For this review, take the finished solid that the model builds, in its own axes (mm). Face numbers are marked on the shaded views. A direction names the side the tool comes from. Coordinates: 2 decimals unless noted, no trailing zeros. Order: outer loops, then holes, each group sorted by start corner. A loop starts at its lowest first (then second) coordinate and runs counter-clockwise, first axis right, second up.
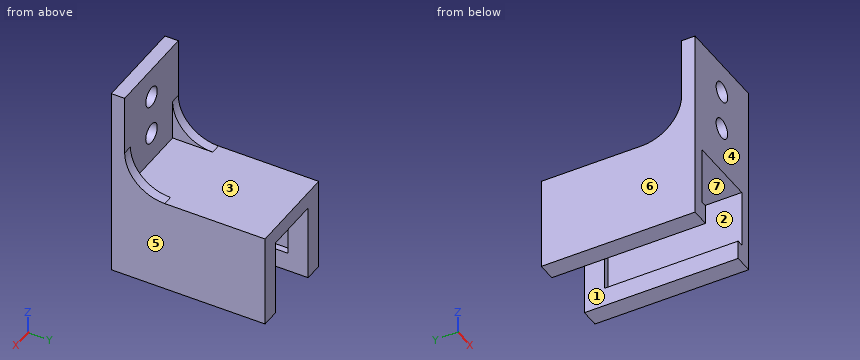
from build123d import *

# Parameters (mm, degrees)
SKETCH1_W           = 14
SKETCH1_H           = 23
BOSS_EXTRUDE1_DEPTH = 14
SKETCH2_W           = 10.4
SKETCH2_H           = 8.65
SKETCH2_W_2         = 8.5
SKETCH2_H_2         = 2.85
CUT_EXTRUDE1_DEPTH  = 20
SKETCH3_W           = 14
SKETCH3_H           = 15
SKETCH3_R           = 1.5
BOSS_EXTRUDE2_DEPTH = 2
BOSS_EXTRUDE3_DEPTH = 1.5
SKETCH5_W           = 8.5
SKETCH5_H           = 11.5
CUT_EXTRUDE2_DEPTH  = 4


with BuildPart() as part:
    # Sketch1 → Boss-Extrude1 (new body)
    with BuildSketch(Plane.XY):
        Rectangle(SKETCH1_W, SKETCH1_H)
    extrude(amount=BOSS_EXTRUDE1_DEPTH)

    # Sketch2 → Cut-Extrude1 (cut)
    with BuildSketch(Plane.XZ.offset(11.5)):
        with Locations((0, 7.175)):
            Rectangle(SKETCH2_W, SKETCH2_H)
        with Locations((0, 1.425)):
            Rectangle(SKETCH2_W_2, SKETCH2_H_2)
    extrude(amount=-CUT_EXTRUDE1_DEPTH, mode=Mode.SUBTRACT)

    # Sketch3 → Boss-Extrude2 (add)
    with BuildSketch(Plane.XZ.offset(11.5)):
        with Locations((0, 21.5)):
            Rectangle(SKETCH3_W, SKETCH3_H)
        with Locations((0, 18.5)):
            Circle(SKETCH3_R, mode=Mode.SUBTRACT)
        with Locations((0, 24.5)):
            Circle(SKETCH3_R, mode=Mode.SUBTRACT)
    extrude(amount=-BOSS_EXTRUDE2_DEPTH)

    # Sketch4 → Boss-Extrude3 (add)
    with BuildSketch(Plane.ZY.offset(7)):
        with BuildLine():
            Line((14, -3.5), (14, -9.5))
            Line((14, -9.5), (20, -9.5))
            ThreePointArc((20, -9.5), (15.757359313, -7.742640687), (14, -3.5))
        make_face()
    boss_extrude3 = extrude(amount=-BOSS_EXTRUDE3_DEPTH)

    # Mirror1: Boss-Extrude3 across plane
    add(boss_extrude3.mirror(Plane(origin=(0, 0, 0), x_dir=(0, 0, 1), z_dir=(1, 0, 0))))

    # Sketch5 → Cut-Extrude2 (cut, through all)
    with BuildSketch(Plane.XZ.offset(-8.5)):
        with Locations((0, 5.75)):
            Rectangle(SKETCH5_W, SKETCH5_H)
    extrude(amount=-CUT_EXTRUDE2_DEPTH, mode=Mode.SUBTRACT)


solid = part.part
1. Machinability: for the marked faces 1, 2, 3 and 4, which of the approach directions +Z, -Z, +X, -X, +Y, -Y give a long, thin tool a straight path to every point of the face, cutting with its end or side? Answer none if there is none.
Answer below:
face 1: -Z, +Y, -Y
face 2: -Y
face 3: +Z, +Y
face 4: +Z, -Z, +X, -X, -Y
2. Take a section at A-A, the plane x = 0. Give the boundary of the cut face in (y, z), plus the area to 3 significant figures.
Answer below:
outline: (-11.5, 11.5) - (11.5, 11.5) - (11.5, 14) - (-9.5, 14) - (-9.5, 17) - (-11.5, 17) - close; (-11.5, 20) - (-9.5, 20) - (-9.5, 23) - (-11.5, 23) - close; (-11.5, 26) - (-9.5, 26) - (-9.5, 29) - (-11.5, 29) - close
area: 75.5 mm2
3. Clearance check with flat-ended pins moving along their axes: pin 1 Ø1 at (x, z) = (-4.5, 5.5) entering from -Y; pin 2 Ø0.5 at (x, y) = (4.5, -4) entering from +Z; pin 3 Ø2.5 at (x, z) = (0, 18.5) entering from +Y; pin 4 Ø5 at (x, z) = (5, 18.5) entering from +Y. State where each tip first meets the part, or that it passes through.
Answer below:
pin 1: stops at y = 8.5
pin 2: stops at z = 14
pin 3: passes through
pin 4: stops at y = -8.02
4. Take a section at C-C, the plane y = -10. Give the boundary of the cut face in (x, z).
Answer below:
outline: (-7, 0) - (-4.25, 0) - (-4.25, 2.85) - (-5.2, 2.85) - (-5.2, 11.5) - (5.2, 11.5) - (5.2, 2.85) - (4.25, 2.85) - (4.25, 0) - (7, 0) - (7, 29) - (-7, 29) - close; hole circle Ø3 at (0, 18.5); hole circle Ø3 at (0, 24.5)
5. Take a section at B-B, the plane z = 24.5. Give the boundary of the cut face in (x, y).
Answer below:
outline: (-7, -11.5) - (-1.5, -11.5) - (-1.5, -9.5) - (-7, -9.5) - close; (1.5, -11.5) - (7, -11.5) - (7, -9.5) - (1.5, -9.5) - close
6. Take a section at D-D, the plane y = 1.25. Give the boundary of the cut face in (x, z), plus the area to 3 significant figures.
Answer below:
outline: (-7, 0) - (-4.25, 0) - (-4.25, 2.85) - (-5.2, 2.85) - (-5.2, 11.5) - (5.2, 11.5) - (5.2, 2.85) - (4.25, 2.85) - (4.25, 0) - (7, 0) - (7, 14) - (-7, 14) - close
area: 81.8 mm2
7. The part is to be moulded in two halves that separate along X. For the marked faces 5, 6 and 7, say which applies: +X half, -X half, draft (parallel to the pull), parting line (faces both ways), or undercut.
Answer below:
face 5: +X half
face 6: -X half
face 7: undercut
8. To check wall thickness, follow L1, parallel to Z at x = 0, y = -10.9; L2, parallel to X at y = 3, z = 4.5; L3, parallel to Y at x = -4.75, z = 20.5. State the ranges of each line that lie inside material, in increasing order.
Answer below:
L1: z = 11.5 to 17, 20 to 23, 26 to 29
L2: x = -7 to -5.2, 5.2 to 7
L3: y = -11.5 to -9.5
